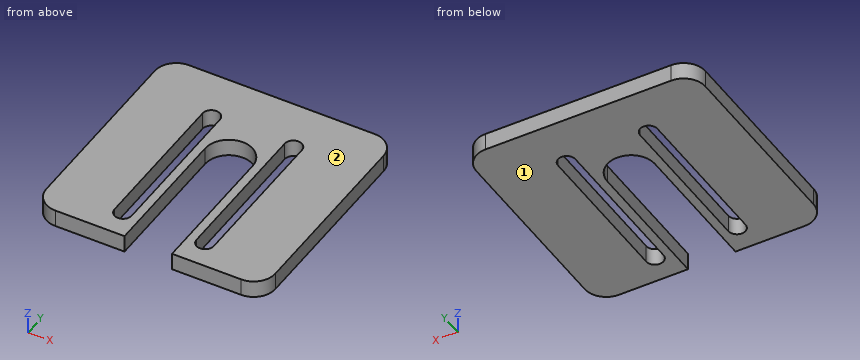
from build123d import *

# Parameters (mm, degrees)
BOSS_EXTRUDE2_DEPTH = 4


with BuildPart() as part:
    # Sketch1 → Boss-Extrude2 (new body)
    with BuildSketch(Plane.XY):
        with BuildLine():
            Line((0, 48), (0, 5))
            ThreePointArc((0, 5), (1.464466094, 1.464466094), (5, 0))
            Line((5, 0), (21, 0))
            Line((21, 0), (21, 31.99499657))
            ThreePointArc((21, 31.99499657), (26.5, 37.49499657), (32, 31.99499657))
            Line((32, 31.99499657), (32, 0))
            Line((32, 0), (48, 0))
            ThreePointArc((48, 0), (51.535533906, 1.464466094), (53, 5))
            Line((53, 5), (53, 48))
            ThreePointArc((53, 48), (51.535533906, 51.535533906), (48, 53))
            Line((48, 53), (5, 53))
            ThreePointArc((5, 53), (1.464466094, 51.535533906), (0, 48))
        make_face()
        with BuildLine():
            Line((19, 41.300206215), (19, 6.300206215))
            ThreePointArc((19, 6.300206215), (17, 4.300206215), (15, 6.300206215))
            Line((15, 6.300206215), (15, 41.300206215))
            ThreePointArc((15, 41.300206215), (17, 43.300206215), (19, 41.300206215))
        make_face(mode=Mode.SUBTRACT)
        with BuildLine():
            Line((38, 41.300206215), (38, 6.300206215))
            ThreePointArc((38, 6.300206215), (36, 4.300206215), (34, 6.300206215))
            Line((34, 6.300206215), (34, 41.300206215))
            ThreePointArc((34, 41.300206215), (36, 43.300206215), (38, 41.300206215))
        make_face(mode=Mode.SUBTRACT)
    extrude(amount=BOSS_EXTRUDE2_DEPTH)


solid = part.part
The model under review builds one solid part; all positions refer to its coordinate system, in mm. Face numbers are marked on the shaded views. Coordinates: 2 decimals unless noted, no trailing zeros. Loops run counter-clockwise (first coordinate to the right, second up) from the corner with the lowest first, then second, coordinate; pieces in that order, holes last.
(1) Consider section B-B, the plane y = 40.5. Give the boundary of the cut face in (x, z).
Determined:
outline: (0, 0) - (15, 0) - (15, 4) - (0, 4) - close; (19, 0) - (34, 0) - (34, 4) - (19, 4) - close; (38, 0) - (53, 0) - (53, 4) - (38, 4) - close
(2) Consider section C-C, the plane x = 36. Give the boundary of the cut face in (y, z), plus the area to 3 significant figures.
Determined:
outline: (0, 0) - (4.3, 0) - (4.3, 4) - (0, 4) - close; (43.3, 0) - (53, 0) - (53, 4) - (43.3, 4) - close
area: 56.0 mm2
(3) Consider section D-D, the plane z = 2.1. Give the boundary of the cut face in (x, y) (3 decimals), plus the area to 3 significant figures.
Determined:
outline: (0, 5) arc R5 ccw to (5, 0) - (21, 0) - (21, 31.995) arc R5.5 cw to (32, 31.995) - (32, 0) - (48, 0) arc R5 ccw to (53, 5) - (53, 48) arc R5 ccw to (48, 53) - (5, 53) arc R5 ccw to (0, 48) - close; hole (15, 6.3) arc R2 ccw to (19, 6.3) - (19, 41.3) arc R2 ccw to (15, 41.3) - close; hole (34, 6.3) arc R2 ccw to (38, 6.3) - (38, 41.3) arc R2 ccw to (34, 41.3) - close
area: 2,080 mm2
(4) Draft analysis for pull direction Z (two halves, no side actions). For the marked faces 1 and 2, state which applies: +Z half, -Z half, draft (parallel to the pull), parting line (faces both ways), or undercut.
Determined:
face 1: -Z half
face 2: +Z half
(5) Insertion check: P1, Ø12, axis at x = 17, y = 26, coming from the -Z side. The pin has a flat end and moves straight along its axis. Give the tip position at first contact, or say it passes through.
Determined:
P1: stops at z = 0
(6) Wall thickness on L1, parallel to X at y = 16, z = 0.4; L2, parallel to X at y = 39, z = 1.35; L3, parallel to X at y = 35.5, z = 2.2: over which ranges is each line inside the solid? List them lowest first.
Determined:
L1: x = 0 to 15, 19 to 21, 32 to 34, 38 to 53
L2: x = 0 to 15, 19 to 34, 38 to 53
L3: x = 0 to 15, 19 to 22.26, 30.74 to 34, 38 to 53
(7) Consider section A-A, the plane y = 31. Give the boundary of the cut face in (x, z).
Determined:
outline: (0, 0) - (15, 0) - (15, 4) - (0, 4) - close; (19, 0) - (21, 0) - (21, 4) - (19, 4) - close; (32, 0) - (34, 0) - (34, 4) - (32, 4) - close; (38, 0) - (53, 0) - (53, 4) - (38, 4) - close
